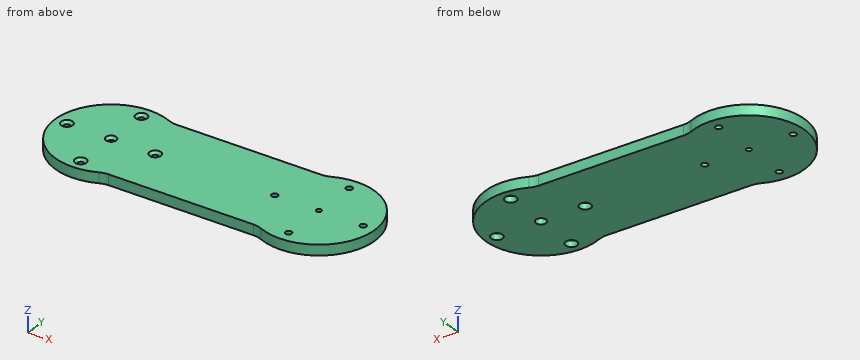
from build123d import *

# Parameters (mm, degrees)
EXTRUDE_1_DEPTH     = 10
FILLET_1_R          = 20
SKETCH_2_R          = 3
SKETCH_2_R_2        = 2.5
CUT_EXTRUDE_1_DEPTH = 10
SKETCH_3_R          = 5.5
SKETCH_3_R_2        = 5
CUT_EXTRUDE_2_DEPTH = 6
SKETCH_4_R          = 2.5
CUT_EXTRUDE_3_DEPTH = 10
SKETCH_5_R          = 3
CUT_EXTRUDE_4_DEPTH = 10
CHAMFER_1_SIZE      = 2.5


with BuildPart() as part:
    # Эскиз1 → Бобышка-Вытянуть1 (new body)
    with BuildSketch(Plane.XY):
        with BuildLine():
            Line((-49.694865317, 47.5), (98.933936526, 47.5))
            ThreePointArc((98.933936526, 47.5), (178.619535605, 0), (98.933936526, -47.5))
            Line((98.933936526, -47.5), (-49.694865317, -47.5))
            ThreePointArc((-49.694865317, -47.5), (-129.380464395, 0), (-49.694865317, 47.5))
        make_face()
    extrude(amount=EXTRUDE_1_DEPTH)

    # Скругление1
    fillet_1_edges = [part.edges().sort_by_distance(p)[0] for p in [
        (-49.694865317, 47.5, 5),
        (98.933936526, 47.5, 5),
        (98.933936526, -47.5, 5),
        (-49.694865317, -47.5, 5),
    ]]
    fillet(fillet_1_edges, radius=FILLET_1_R)

    # Эскиз2 → Вырез-Вытянуть1 (cut)
    with BuildSketch(Plane(origin=(0, 0, 0), x_dir=(-1, 0, 0), z_dir=(0, 0, -1))):
        with Locations((-124.619535605, 42.5)):
            Circle(SKETCH_2_R)
        with Locations((-124.619535605, -42.5)):
            Circle(SKETCH_2_R)
        with Locations((-82.119535605, 0)):
            Circle(SKETCH_2_R)
        with Locations((-167.119535605, 0)):
            Circle(SKETCH_2_R)
        with Locations((-124.619535605, 0)):
            Circle(SKETCH_2_R_2)
    extrude(amount=-CUT_EXTRUDE_1_DEPTH, mode=Mode.SUBTRACT)

    # Эскиз3 → Вырез-Вытянуть2 (cut)
    with BuildSketch(Plane(origin=(0, 0, 0), x_dir=(-1, 0, 0), z_dir=(0, 0, -1))):
        with Locations((-124.619535605, 42.5)):
            Circle(SKETCH_3_R)
        with Locations((-167.119535605, 0)):
            Circle(SKETCH_3_R)
        with Locations((-124.619535605, -42.5)):
            Circle(SKETCH_3_R)
        with Locations((-82.119535605, 0)):
            Circle(SKETCH_3_R)
        with Locations((-124.619535605, 0)):
            Circle(SKETCH_3_R_2)
    extrude(amount=-CUT_EXTRUDE_2_DEPTH, mode=Mode.SUBTRACT)

    # Эскиз4 → Вырез-Вытянуть3 (cut)
    with BuildSketch(Plane(origin=(0, 0, 0), x_dir=(-1, 0, 0), z_dir=(0, 0, -1))):
        with Locations((75.380464395, 0)):
            Circle(SKETCH_4_R)
    extrude(amount=-CUT_EXTRUDE_3_DEPTH, mode=Mode.SUBTRACT)

    # Эскиз5 → Вырез-Вытянуть4 (cut)
    with BuildSketch(Plane(origin=(0, 0, 0), x_dir=(-1, 0, 0), z_dir=(0, 0, -1))):
        with Locations((75.380464395, 42.5)):
            Circle(SKETCH_5_R)
        with Locations((75.380464395, -42.5)):
            Circle(SKETCH_5_R)
        with Locations((32.880464395, 0)):
            Circle(SKETCH_5_R)
        with Locations((117.880464395, 0)):
            Circle(SKETCH_5_R)
    extrude(amount=-CUT_EXTRUDE_4_DEPTH, mode=Mode.SUBTRACT)

    # Фаска1
    chamfer_1_edges = [part.edges().sort_by_distance(p)[0] for p in [
        (-72.380464395, -42.5, 10),
        (-29.880464395, 0, 10),
        (-114.880464395, 0, 10),
        (-72.880464395, 0, 10),
        (-72.380464395, 42.5, 10),
    ]]
    chamfer(chamfer_1_edges, length=CHAMFER_1_SIZE)


solid = part.part
CAD build for the part. Positions are in the model's coordinates, mm. Give positions to 0.01 mm unless a question says otherwise; leave off trailing zeros. Order: outer loops, then holes, each group sorted by start corner. A loop starts at its lowest first (then second) coordinate and runs counter-clockwise, first axis right, second up. Notation, with made-up numbers: (-29, -36) - (16, -36) arc R27 ccw to (16, -3) - close; hole circle Ø4 at (-1, 30.25). An arc over 180 degrees is marked (long way). Write each question's results on one line, items separated by ' | '.
1. Saw through at A-A on z = 2. Count the separate pieces of the cut face and the enclosed holes in it, and give its area (3 significant figures).
Calculated:
separate pieces: 1 | enclosed holes: 10 | area: 28,000 mm2
2. Pin check, flat tips, straight feed: pin 1 (5 mm diameter, centred on y = -26, z = 5, fed in from +X); pin 2 (5.5 mm diameter, centred on x = -117.88, y = 0, fed in from +Z); pin 3 (3.5 mm diameter, centred on x = 81, y = -2, fed in from -Z); pin 4 (6.5 mm diameter, centred on x = -75.38, y = 0, fed in from +Z). Stop position of each tip, or through.
Calculated:
pin 1: stops at x = 173.24 | pin 2: passes through | pin 3: stops at z = 6 | pin 4: stops at z = 8.25
3. Probe L1, parallel to X at y = 40.5, z = 2.75; L2, parallel to X at y = -43, z = 2.25; L3, parallel to Y at x = 21, z = 6. List the from-to ranges inside material, lowest first. Write a range as from..to.
Calculated:
L1: x = -111.1..-77.62, -73.14..119.5, 129.74..160.34 | L2: x = -108.05..-78.34, -72.42..119.14, 130.1..157.28 | L3: y = -47.5..47.5
4. Saw through at B-B on y = -42.5. List the corners of the cut face in (x, z), and give its area (3 significant figures).
Calculated:
outline: (-108.69, 0) - (-78.38, 0) - (-78.38, 7.5) - (-80.88, 10) - (-108.69, 10) - close; (-72.38, 0) - (119.12, 0) - (119.12, 6) - (121.62, 6) - (121.62, 10) - (-69.88, 10) - (-72.38, 7.5) - close; (127.62, 6) - (130.12, 6) - (130.12, 0) - (157.93, 0) - (157.93, 10) - (127.62, 10) - close | area: 2,510 mm2
5. Saw through at D-D on y = 30.5. List the corners of the cut face in (x, z).
Calculated:
outline: (-119.94, 0) - (169.18, 0) - (169.18, 10) - (-119.94, 10) - close
6. Saw through at C-C on x = 2.5. List the corners of the cut face in (y, z).
Calculated:
outline: (-47.5, 0) - (47.5, 0) - (47.5, 10) - (-47.5, 10) - close
